Can you work these out from the model? Positions are in its coordinate system, mm. Face numbers are marked on the shaded views. A direction names the side the tool comes from. Coordinates: 2 decimals unless noted, no trailing zeros. Order: outer loops, then holes, each group sorted by start corner. A loop starts at its lowest first (then second) coordinate and runs counter-clockwise, first axis right, second up. Notation, with made-up numbers: (70, 26) - (105, 26) arc R14 cw to (105, 46) - close; hole circle Ø9 at (63, 13.5). An arc over 180 degrees is marked (long way). Return JSON: item names as keys, results as strings. Group by question number.
1) Imagine slicing it at B-B (x = 0). Write out the boundary of the cut face in (y, z).
2) Imagine slicing it at D-D (y = 8). Write out the boundary of the cut face in (x, z), and give its area (3 significant figures).
3) If I drill on line 1 along Z through (x, y) = (13.1, 0); line 2 along X through (y, z) = (-1, -10.5); line 3 along Y through (x, z) = (-13.4, 0), over which ranges is the centre line in solid material (lowest first)?
4) Imagine slicing it at A-A (x = 8). Write out the boundary of the cut face in (y, z).
5) Imagine slicing it at C-C (z = 8). Write out the boundary of the cut face in (x, y), and give its area (3 significant figures).
6) For pin 1 Ø6 at (x, z) = (-4.5, -3) entering from +Y; pin 2 Ø8 at (x, z) = (11, -11) entering from +Y, each with a flat end and sliding along its axis, tell me the tip position at first contact or that it passes through.
7) Which directions (+Z, -Z, +X, -X, +Y, -Y) give clear straight access to the entire face, cutting with the end or side of a thin tool? Please do the marked faces 4 and 5.
8) If we mould it in two halves opening along X, with no side actions, what happens to the marked faces 1, 2 and 3? For each: pulls with the +X half, pulls with the -X half, needs draft (parallel to the pull), parting line crosses it, or undercut.
```python
from build123d import *

# Parameters (mm, degrees)
SKETCH1_R                = 4
SKETCH1_R_2              = 1.85
BOSS_EXTRUDE1_DEPTH      = 14
BOSS_EXTRUDE1_DEPTH_BACK = 14
CUT_EXTRUDE1_DEPTH       = 12
CUT_EXTRUDE1_DEPTH_BACK  = 12
SKETCH3_R                = 4
SKETCH3_R_2              = 1.85
CUT_EXTRUDE2_DEPTH       = 2
FILLET1_R                = 2.5


with BuildPart() as part:
    # Sketch1 → Boss-Extrude1 (new body, two sides)
    with BuildSketch(Plane(origin=(0, 0, 0), x_dir=(0, 0, -1), z_dir=(1, 0, 0))) as boss_extrude1_sk:
        with BuildLine():
            Line((-14, 0), (-14, -16))
            Line((-14, -16), (14, -16))
            Line((14, -16), (14, 0))
            ThreePointArc((14, 0), (0, 14), (-14, 0))
        make_face()
        Circle(SKETCH1_R, mode=Mode.SUBTRACT)
        with Locations((0, 8)):
            Circle(SKETCH1_R_2, mode=Mode.SUBTRACT)
        with Locations((5.656854249, 5.656854249)):
            Circle(SKETCH1_R_2, mode=Mode.SUBTRACT)
        with Locations((8, 0)):
            Circle(SKETCH1_R_2, mode=Mode.SUBTRACT)
        with Locations((5.656854249, -5.656854249)):
            Circle(SKETCH1_R_2, mode=Mode.SUBTRACT)
        with Locations((0, -8)):
            Circle(SKETCH1_R_2, mode=Mode.SUBTRACT)
        with Locations((-5.656854249, -5.656854249)):
            Circle(SKETCH1_R_2, mode=Mode.SUBTRACT)
        with Locations((-8, 0)):
            Circle(SKETCH1_R_2, mode=Mode.SUBTRACT)
        with Locations((-5.656854249, 5.656854249)):
            Circle(SKETCH1_R_2, mode=Mode.SUBTRACT)
    extrude(amount=BOSS_EXTRUDE1_DEPTH)
    extrude(boss_extrude1_sk.sketch, amount=-BOSS_EXTRUDE1_DEPTH_BACK)

    # Sketch2 → Cut-Extrude1 (cut, two sides)
    with BuildSketch(Plane(origin=(0, 0, 0), x_dir=(0, 0, -1), z_dir=(1, 0, 0))) as cut_extrude1_sk:
        with BuildLine():
            Line((-14, 0), (-14, -14))
            Line((-14, -14), (14, -14))
            Line((14, -14), (14, 0))
            ThreePointArc((14, 0), (0, 14), (-14, 0))
        make_face()
    extrude(amount=CUT_EXTRUDE1_DEPTH, mode=Mode.SUBTRACT)
    extrude(cut_extrude1_sk.sketch, amount=-CUT_EXTRUDE1_DEPTH_BACK, mode=Mode.SUBTRACT)

    # Sketch3 → Cut-Extrude2 (cut)
    with BuildSketch(Plane.XZ.offset(16)):
        Circle(SKETCH3_R)
        with Locations((0, 8)):
            Circle(SKETCH3_R_2)
        with Locations((5.656854249, 5.656854249)):
            Circle(SKETCH3_R_2)
        with Locations((8, 0)):
            Circle(SKETCH3_R_2)
        with Locations((5.656854249, -5.656854249)):
            Circle(SKETCH3_R_2)
        with Locations((0, -8)):
            Circle(SKETCH3_R_2)
        with Locations((-5.656854249, -5.656854249)):
            Circle(SKETCH3_R_2)
        with Locations((-8, 0)):
            Circle(SKETCH3_R_2)
        with Locations((-5.656854249, 5.656854249)):
            Circle(SKETCH3_R_2)
    extrude(amount=-CUT_EXTRUDE2_DEPTH, mode=Mode.SUBTRACT)

    # Fillet1
    fillet1_edges = [part.edges().sort_by_distance(p)[0] for p in [
        (-14, -16, 0),
        (14, -16, 0),
    ]]
    fillet(fillet1_edges, radius=FILLET1_R)


solid = part.part
```
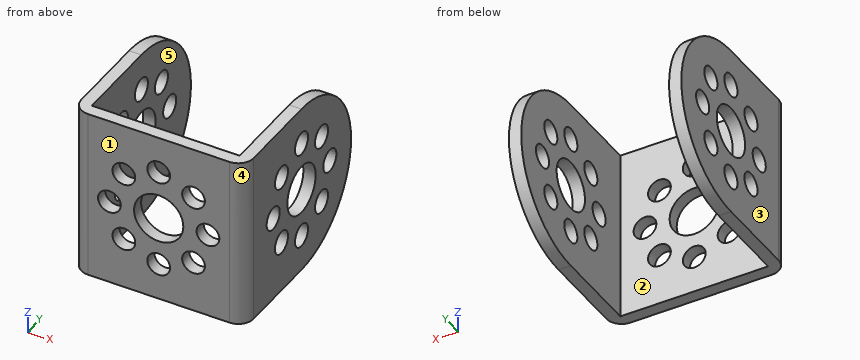
Calculated:
{
 "1": {"outline": "(-16, -14) - (-14, -14) - (-14, -9.85) - (-16, -9.85) - close; (-16, -6.15) - (-14, -6.15) - (-14, -4) - (-16, -4) - close; (-16, 4) - (-14, 4) - (-14, 6.15) - (-16, 6.15) - close; (-16, 9.85) - (-14, 9.85) - (-14, 14) - (-16, 14) - close"},
 "2": {"outline": "(-14, -11.49) - (-12, -11.49) - (-12, -1.85) - (-14, -1.85) - close; (-14, 1.85) - (-12, 1.85) - (-12, 11.49) - (-14, 11.49) - close; (12, -11.49) - (14, -11.49) - (14, -1.85) - (12, -1.85) - close; (12, 1.85) - (14, 1.85) - (14, 11.49) - (12, 11.49) - close", "area": "77.1 mm2"},
 "3": {"line 1": "-14 to -9.85, -6.15 to -4, 4 to 6.15, 9.85 to 14", "line 2": "-14 to -12, 12 to 14", "line 3": "-15.12 to -9.85, -6.15 to -4, 4 to 6.15, 9.85 to 14"},
 "4": {"outline": "(-16, -14) - (-14, -14) - (-14, -1.85) - (-16, -1.85) - close; (-16, 1.85) - (-14, 1.85) - (-14, 14) - (-16, 14) - close"},
 "5": {"outline": "(-14, -13.5) arc R2.5 ccw to (-11.5, -16) - (-1.85, -16) - (-1.85, -14) - (-12, -14) - (-12, -1.85) - (-14, -1.85) - close; (-14, 1.85) - (-12, 1.85) - (-12, 11.49) - (-14, 11.49) - close; (1.85, -16) - (11.5, -16) arc R2.5 ccw to (14, -13.5) - (14, -1.85) - (12, -1.85) - (12, -14) - (1.85, -14) - close; (12, 1.85) - (14, 1.85) - (14, 11.49) - (12, 11.49) - close", "area": "133 mm2"},
 "6": {"pin 1": "y = -14", "pin 2": "y = 12.05"},
 "7": {"face 4": "+Z, -Z, +X, -Y", "face 5": "+Z, -Z, +Y"},
 "8": {"face 1": "needs draft", "face 2": "undercut", "face 3": "pulls with the -X half"}
}
